```python
from build123d import *

# Parameters (mm, degrees)
SKETCH1_W           = 71
SKETCH1_H           = 50.5
SKETCH1_R           = 1
SKETCH1_W_2         = 59
SKETCH1_H_2         = 38.5
BOSS_EXTRUDE1_DEPTH = 3
SKETCH2_R           = 3
SKETCH2_R_2         = 1
BOSS_EXTRUDE2_DEPTH = 2
FILLET1_R           = 3


with BuildPart() as part:
    # Sketch1 → Boss-Extrude1 (new body)
    with BuildSketch(Plane(origin=(0, 0, 0), x_dir=(1, 0, 0), z_dir=(0, 1, 0))):
        Rectangle(SKETCH1_W, SKETCH1_H)
        with Locations(Location((-32.5, 22, 0), (0, 0, 270))):
            Circle(SKETCH1_R, mode=Mode.SUBTRACT)
        with Locations(Location((-32.5, -22, 0), (0, 0, 270))):
            Circle(SKETCH1_R, mode=Mode.SUBTRACT)
        with Locations(Location((32.5, -22, 0), (0, 0, 270))):
            Circle(SKETCH1_R, mode=Mode.SUBTRACT)
        with Locations(Location((32.5, 22, 0), (0, 0, 270))):
            Circle(SKETCH1_R, mode=Mode.SUBTRACT)
        Rectangle(SKETCH1_W_2, SKETCH1_H_2, mode=Mode.SUBTRACT)
    extrude(amount=BOSS_EXTRUDE1_DEPTH)

    # Sketch2 → Boss-Extrude2 (add)
    # profile 1 of 4: a face of its own
    with BuildSketch(Plane(origin=(0, 3, 0), x_dir=(1, 0, 0), z_dir=(0, 1, 0))):
        with Locations((32.5, 22)):
            Circle(SKETCH2_R)
        with Locations(Location((32.5, 22, 0), (0, 0, 270))):
            Circle(SKETCH2_R_2, mode=Mode.SUBTRACT)
    # profile 2 of 4: a face of its own
    with BuildSketch(Plane(origin=(0, 3, 0), x_dir=(1, 0, 0), z_dir=(0, 1, 0))):
        with Locations((32.5, -22)):
            Circle(SKETCH2_R)
        with Locations(Location((32.5, -22, 0), (0, 0, 270))):
            Circle(SKETCH2_R_2, mode=Mode.SUBTRACT)
    # profile 3 of 4: a face of its own
    with BuildSketch(Plane(origin=(0, 3, 0), x_dir=(1, 0, 0), z_dir=(0, 1, 0))):
        with Locations(Location((-32.5, -22, 0), (0, 0, 180))):
            Circle(SKETCH2_R)
        with Locations(Location((-32.5, -22, 0), (0, 0, 270))):
            Circle(SKETCH2_R_2, mode=Mode.SUBTRACT)
    # profile 4 of 4: a face of its own
    with BuildSketch(Plane(origin=(0, 3, 0), x_dir=(1, 0, 0), z_dir=(0, 1, 0))):
        with Locations(Location((-32.5, 22, 0), (0, 0, 180))):
            Circle(SKETCH2_R)
        with Locations(Location((-32.5, 22, 0), (0, 0, 270))):
            Circle(SKETCH2_R_2, mode=Mode.SUBTRACT)
    extrude(amount=BOSS_EXTRUDE2_DEPTH)

    # Fillet1
    fillet1_edges = [part.edges().sort_by_distance(p)[0] for p in [
        (35.5, 1.5, 25.25),
        (-35.5, 1.5, 25.25),
        (-35.5, 1.5, -25.25),
        (35.5, 1.5, -25.25),
    ]]
    fillet(fillet1_edges, radius=FILLET1_R)


solid = part.part
```
Part model, mm, in its own coordinate system. A direction names the side the tool comes from. Round coordinates to 2 decimals unless told otherwise and drop trailing zeros. Write each loop counter-clockwise with the first axis right and the second up, starting at its lowest first coordinate (ties: lowest second). Pieces come first, ordered by that corner, then holes. Notation, with made-up numbers: (16, 47) -> (44, 47) arc R30 cw to (44, 78) -> close; hole circle Ø5 at (-19, 78.25). An arc over 180 degrees is marked (long way). Return JSON: item names as keys, results as strings. Group by question number.
Q1. Mould opens along Z. For faces 4 (the cylindrical face through (-31.51, 2.46, 21.87)), 5 (the flat face through (0, 1, 19.25)), 6 (the flat face through (-35.5, 1, 0)), 7 (the cylindrical face through (-34.6, 1.52, -24.39)) say: pulls with the +Z half, pulls with the -Z half, needs draft (parallel to the pull), parting line crosses it, or undercut.
Q2. Probe L1, parallel to X at y = 2.5, z = 22; L2, parallel to Z at x = -10, y = 1.95; L3, parallel to X at y = 2.1, z = -1.5. List the from-to ranges inside material, lowest first. Write a range as [from, to].
Q3. Saw through at B-B on x = -22.5. Write the cut outline in (y, z), plus the area to 3 significant figures.
Q4. Pin check, flat tip, straight feed: pin 1 (3 mm diameter, centred on x = -32.5, z = -22, fed in from +Y). Stop position of the tip, or through.
Q5. Saw through at A-A on y = 3.75. Write the cut outline in (x, z).
Q6. Which spindle directions (+Z, -Z, +X, -X, +Y, -Y) get a long thin tool onto all of the face, cutting with end or side? Do faces 1 (the flat face through (-34, 5, -22)), 2 (the flat face through (29.5, 1, 0)), 3 (the cylindrical face through (29.5, 4, -22.1)). Say none if no direction does.
Q7. Saw through at C-C on z = 18. Write the cut outline in (x, y).
Answer:
{
 "1": {"face 4": "undercut", "face 5": "undercut", "face 6": "needs draft", "face 7": "pulls with the -Z half"},
 "2": {"L1": "[-35.5, -33.5], [-31.5, 31.5], [33.5, 35.5]", "L2": "[-25.25, -19.25], [19.25, 25.25]", "L3": "[-35.5, -29.5], [29.5, 35.5]"},
 "3": {"outline": "(0, -25.25) -> (3, -25.25) -> (3, -19.25) -> (0, -19.25) -> close; (0, 19.25) -> (3, 19.25) -> (3, 25.25) -> (0, 25.25) -> close", "area": "36.0 mm2"},
 "4": {"pin 1": "y = 5"},
 "5": {"outline": "circle Ø6 at (-32.5, -22); circle Ø6 at (-32.5, 22); circle Ø6 at (32.5, -22); circle Ø6 at (32.5, 22); hole circle Ø2 at (-32.5, -22); hole circle Ø2 at (-32.5, 22); hole circle Ø2 at (32.5, -22); hole circle Ø2 at (32.5, 22)"},
 "6": {"face 1": "+Z, -Z, +X, -X, +Y", "face 2": "+Y, -Y", "face 3": "+Y"},
 "7": {"outline": "(-35.5, 0) -> (-29.5, 0) -> (-29.5, 3) -> (-35.5, 3) -> close; (29.5, 0) -> (35.5, 0) -> (35.5, 3) -> (29.5, 3) -> close"}
}
